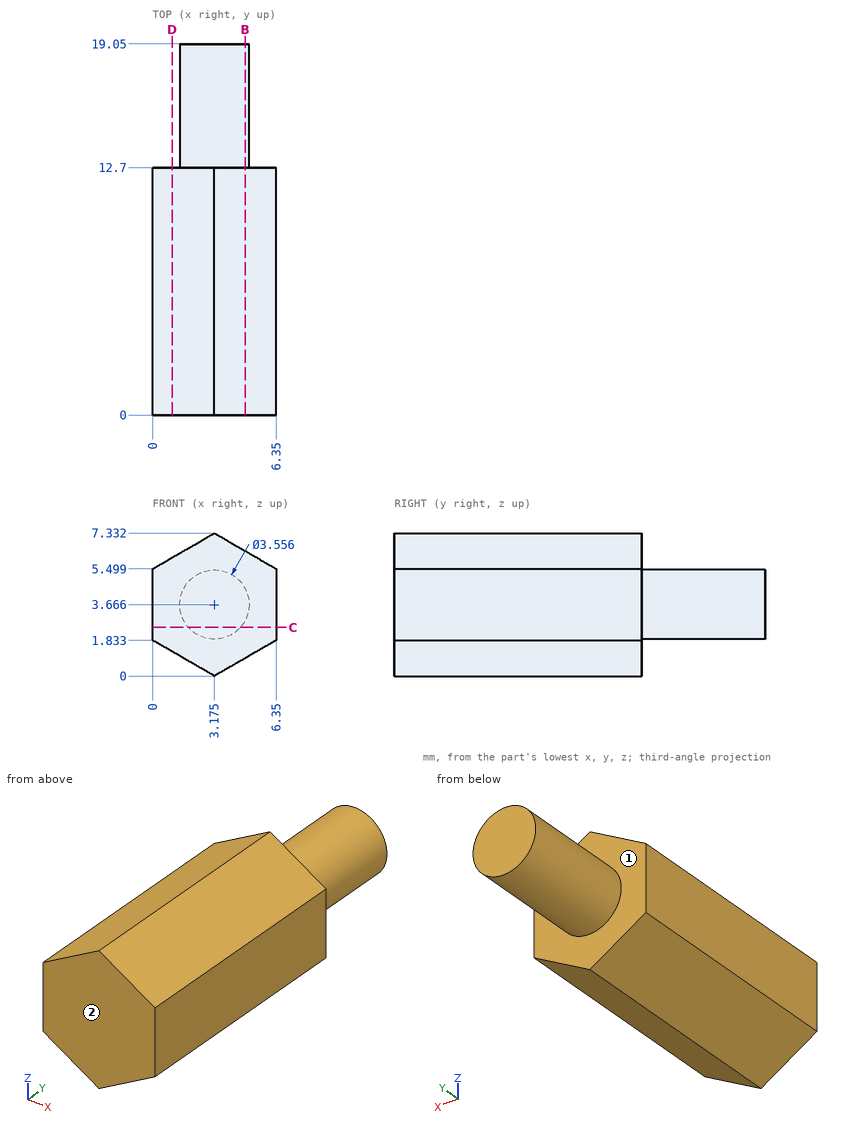
Can you work these out from the drawing? Everything is in mm from the part's minimum corner. A direction names the side the tool comes from. Coordinates: 2 decimals unless noted, no trailing zeros. Order: outer loops, then holes, each group sorted by start corner. A loop starts at its lowest first (then second) coordinate and runs counter-clockwise, first axis right, second up. Notation, with made-up numbers: M -14.75,50.25 L 26.25,50.25 A5 ccw 26.25,56.25 Z; hole C -33.75,-15.75 d11. An arc over 180 degrees is marked long. Answer as CSV lines item,"result". Start each with the question number.
1. I need wall thicknesses on line 1 (Y direction, x = 5.5, z = 2.5); line 2 (Z direction, x = 3.25, y = 15.5); line 3 (Z direction, x = 3.75, y = 9.75). Which ranges of each line are inside material? Lowest first, please. Write a range as [from, to].
2. For pin 1 (2 mm diameter, centred on x = 1.5, y = 4, fed in from -Z), with a flat end and sliding along its axis, tell me the tip position at first contact or that it passes through.
3. I want a section at D-D, the plane x = 1. Write out the boundary of the cut face in (y, z).
4. I want a section at C-C, the plane z = 2.5. Write out the boundary of the cut face in (x, y).
5. I want a section at B-B, the plane x = 4.75. Write out the boundary of the cut face in (y, z), and give its area (3 significant figures).
6. On a 3-axis mill with a long thin cutter (end or side, diameter ignored), from which of +Z, -Z, +X, -X, +Y, -Y can I reach the whole of each face in a straight line? I mean the marked faces 1 and 2. Say none if no direction works.
Recorded:
1,line 1,"y = [0, 12.7]"
1,line 2,"z = [1.89, 5.44]"
1,line 3,"z = [0.33, 7]"
2,pin 1,"stops at z = 0.39"
3,outline,"M 0,1.26 L 12.7,1.26 L 12.7,6.08 L 0,6.08 Z"
4,outline,"M 0,0 L 6.35,0 L 6.35,12.7 L 4.52,12.7 L 4.52,19.05 L 1.83,19.05 L 1.83,12.7 L 0,12.7 Z"
5,outline,"M 0,0.91 L 12.7,0.91 L 12.7,2.84 L 19.05,2.84 L 19.05,4.49 L 12.7,4.49 L 12.7,6.42 L 0,6.42 Z"
5,area,"80.5 mm2"
6,face 1,"+Y"
6,face 2,"+Z, -Z, +X, -X, -Y"
